Geometry: final body of the model. Coordinates: model frame, mm. A direction names the side the tool comes from. Coordinates: 2 decimals unless noted, no trailing zeros. Write each loop counter-clockwise with the first axis right and the second up, starting at its lowest first coordinate (ties: lowest second). Pieces come first, ordered by that corner, then holes. Notation, with made-up numbers: (34.5, -20.75) -> (62.5, -20.75) arc R20 cw to (62.5, -6.75) -> close; hole circle Ø8 at (14.5, 40). An arc over 180 degrees is marked (long way). Answer as a JSON object with one key per item and string values. Group by question number.
```python
from build123d import *

# Parameters (mm, degrees)
F0_W     = 116.9285327196
F0_H     = 89.5570702851
F1_DEPTH = 92.71
F3_DEPTH = 116.9295327196
F4_W     = 56.9494720548
F4_H     = 39.7882887628
F5_DEPTH = 92.711


with BuildPart() as f1:
    # F0 (on Front) → F1 (new body)
    with BuildSketch(Plane.XZ):
        with Locations((15.2437537909, -1.4810357243)):
            Rectangle(F0_W, F0_H)
    extrude(amount=F1_DEPTH)

    # F2 (on face) → F3 (cut, through all)
    with BuildSketch(Plane(origin=(-43.220512569, 0, 0), x_dir=(0, -1, 0), z_dir=(-1, 0, 0))):
        with BuildLine():
            ThreePointArc((92.71, -25.0020706653), (141.0050891582, -4.9975897399), (161.0095700836, 43.2974994183))
            ThreePointArc((161.0095700836, 43.2974994183), (92.71, 111.5970695018), (24.4104299164, 43.2974994183))
            Line((24.4104299164, 43.2974994183), (92.71, 43.2974994183))
            Line((92.71, 43.2974994183), (92.71, -25.0020706653))
        make_face()
        with BuildLine():
            Line((92.71, 43.2974994183), (24.4104299164, 43.2974994183))
            ThreePointArc((24.4104299164, 43.2974994183), (44.4149108418, -4.9975897399), (92.71, -25.0020706653))
            Line((92.71, -25.0020706653), (92.71, 43.2974994183))
        make_face()
    extrude(amount=-F3_DEPTH, mode=Mode.SUBTRACT)

    # F4 (on face) → F5 (cut, through all)
    with BuildSketch(Plane(origin=(0, 0, 0), x_dir=(-1, 0, 0), z_dir=(0, 1, 0))):
        with Locations((-15.7413156703, 23.4033550369)):
            Rectangle(F4_W, F4_H)
    extrude(amount=-F5_DEPTH, mode=Mode.SUBTRACT)


solid = f1.part
```
Item 1: Set-up query: faces 4 (the flat face through (14, -92.71, -35)), 5 (the flat face through (-12.733, -14, 23)). Return all of +Z, -Z, +X, -X, +Y, -Y with unobstructed straight access to the full face (end or side cutting, diameter ignored); none if empty.
Item 2: Mould query, pull axis X, two halves, no side actions, for faces 1 (the flat face through (-43.221, -35, -12)), 2 (the cylindrical face through (14.4, -52.9, -12.2)), 3 (the flat face through (44.216, -14, 23)). Classes: +X half, -X half, draft (parallel to the pull), parting line (faces both ways), or undercut.
Item 3: Ray query, L1, parallel to X at y = -15, z = 18; L2, parallel to Z at x = 26.5, y = -18; L3, parallel to Z at x = 20, y = -61. Return the intervals inside material, ascending. Write a range as [from, to].
Item 4: Section C-C on z = 34. Output: boundary loops of the cut face in (x, y), then the cut area to 3 significant figures.
Item 5: Section A-A on z = 18.5. Output: boundary loops of the cut face in (x, y).
Item 6: Section B-B on x = -7.5. Output: boundary loops of the cut face in (y, z), then the cut area to 3 significant figures.
Item 7: Contact query for flat-ended pins moving along their axis: pin 1 (18.5 mm diameter, centred on x = 4.5, y = -9.5, fed in from +Z); pin 2 (6 mm diameter, centred on x = 62, y = -52, fed in from +Z); pin 3 (2 mm diameter, centred on x = 17.5, z = -9, fed in from -Y). Output: stop coordinate, or through.
Item 8: Section D-D on y = -66.5. Output: boundary loops of the cut face in (x, z).
Answer sheet:
{
 "1": {"face 4": "+Z, -Z, +X, -X, -Y", "face 5": "+Z, +Y, -Y"},
 "2": {"face 1": "-X half", "face 2": "draft", "face 3": "undercut"},
 "3": {"L1": "x = [-43.22, -12.73], [44.22, 73.71]", "L2": "z = [-46.26, 3.51]", "L3": "z = [-46.26, -17.19]"},
 "4": {"outline": "(-43.22, -25.05) -> (-12.73, -25.05) -> (-12.73, 0) -> (-43.22, 0) -> close; (44.22, -25.05) -> (73.71, -25.05) -> (73.71, 0) -> (44.22, 0) -> close", "area": "1,500 mm^2"},
 "5": {"outline": "(-43.22, -29.07) -> (-12.73, -29.07) -> (-12.73, 0) -> (-43.22, 0) -> close; (44.22, -29.07) -> (73.71, -29.07) -> (73.71, 0) -> (44.22, 0) -> close"},
 "6": {"outline": "(-92.71, -46.26) -> (0, -46.26) -> (0, 3.51) -> (-37.2, 3.51) arc R68.3 cw to (-92.71, -25) -> close", "area": "3,510 mm^2"},
 "7": {"pin 1": "stops at z = 3.51", "pin 2": "stops at z = -9.18", "pin 3": "stops at y = -50"},
 "8": {"outline": "(-43.22, -46.26) -> (73.71, -46.26) -> (73.71, -19.77) -> (-43.22, -19.77) -> close"}
}
